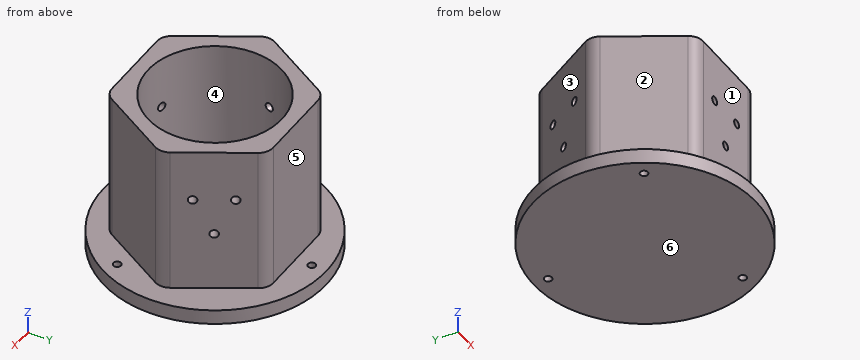
```python
from build123d import *

# Parameters (mm, degrees)
SKETCH1_R               = 75
BOSS_EXTRUDE1_DEPTH     = 10
BOSS_EXTRUDE2_DEPTH     = 100
SKETCH4_R               = 45
CUT_EXTRUDE1_DEPTH      = 100
CUT_EXTRUDE2_REACH      = 187.469
CUT_EXTRUDE2_END_RADIUS = 45
SKETCH5_R               = 2.8
CIRPATTERN1_COUNT       = 3
SKETCH7_R               = 2.55
CUT_EXTRUDE3_DEPTH      = 10


with BuildPart() as part:
    # Sketch1 → Boss-Extrude1 (new body)
    with BuildSketch(Plane.XY):
        Circle(SKETCH1_R)
    extrude(amount=BOSS_EXTRUDE1_DEPTH)

    # Sketch2 → Boss-Extrude2 (add)
    with BuildSketch(Plane.XY.offset(10)):
        with BuildLine():
            Line((59.613248654, 5), (34.136751346, 49.126587737))
            ThreePointArc((34.136751346, 49.126587737), (30.476497308, 52.786841774), (25.476497308, 54.126587737))
            Line((25.476497308, 54.126587737), (-25.476497308, 54.126587737))
            ThreePointArc((-25.476497308, 54.126587737), (-30.476497308, 52.786841774), (-34.136751346, 49.126587737))
            Line((-34.136751346, 49.126587737), (-59.613248654, 5))
            ThreePointArc((-59.613248654, 5), (-60.952994616, 0), (-59.613248654, -5))
            Line((-59.613248654, -5), (-34.136751346, -49.126587737))
            ThreePointArc((-34.136751346, -49.126587737), (-30.476497308, -52.786841774), (-25.476497308, -54.126587737))
            Line((-25.476497308, -54.126587737), (25.476497308, -54.126587737))
            ThreePointArc((25.476497308, -54.126587737), (30.476497308, -52.786841774), (34.136751346, -49.126587737))
            Line((34.136751346, -49.126587737), (59.613248654, -5))
            ThreePointArc((59.613248654, -5), (60.952994616, 0), (59.613248654, 5))
        make_face()
    extrude(amount=BOSS_EXTRUDE2_DEPTH)

    # Sketch4 → Cut-Extrude1 (cut)
    with BuildSketch(Plane.XY.offset(110)):
        Circle(SKETCH4_R)
    extrude(amount=-CUT_EXTRUDE1_DEPTH, mode=Mode.SUBTRACT)

    # Cut-Extrude2: up to this cylinder (the profile starts outside it)
    cut_extrude2_end = Plane(origin=(0, 0, 62.5), z_dir=(0, 0, 1)) * Cylinder(CUT_EXTRUDE2_END_RADIUS, 490.938, mode=Mode.PRIVATE)
    # Sketch5 → Cut-Extrude2 (cut, up to the surface)
    with BuildSketch(Plane.XZ.offset(54.126587737), mode=Mode.PRIVATE) as cut_extrude2_sk1:
        with Locations((0, 50)):
            Circle(SKETCH5_R)
    cut_extrude2_tool1 = extrude(cut_extrude2_sk1.sketch, amount=-CUT_EXTRUDE2_REACH, mode=Mode.PRIVATE) - cut_extrude2_end
    # Sketch5 → Cut-Extrude2 (cut, up to the surface)
    with BuildSketch(Plane.XZ.offset(54.126587737), mode=Mode.PRIVATE) as cut_extrude2_sk2:
        with Locations((-12.5, 75)):
            Circle(SKETCH5_R)
    cut_extrude2_tool2 = extrude(cut_extrude2_sk2.sketch, amount=-CUT_EXTRUDE2_REACH, mode=Mode.PRIVATE) - cut_extrude2_end
    # Sketch5 → Cut-Extrude2 (cut, up to the surface)
    with BuildSketch(Plane.XZ.offset(54.126587737), mode=Mode.PRIVATE) as cut_extrude2_sk3:
        with Locations((12.5, 75)):
            Circle(SKETCH5_R)
    cut_extrude2_tool3 = extrude(cut_extrude2_sk3.sketch, amount=-CUT_EXTRUDE2_REACH, mode=Mode.PRIVATE) - cut_extrude2_end
    cut_extrude2 = cut_extrude2_tool1.solids().sort_by_distance((0, -54.126588, 50))[0] + cut_extrude2_tool2.solids().sort_by_distance((-12.5, -54.126588, 75))[0] + cut_extrude2_tool3.solids().sort_by_distance((12.5, -54.126588, 75))[0]
    add(cut_extrude2, mode=Mode.SUBTRACT)

    # CirPattern1: Cut-Extrude2 ×3 about axis
    cirpattern1_axis = Axis((0, 0, -117.279220614), (0, 0, 1))
    for i in range(1, CIRPATTERN1_COUNT):
        add(cut_extrude2.rotate(cirpattern1_axis, i * 360 / CIRPATTERN1_COUNT), mode=Mode.SUBTRACT)

    # Sketch7 → Cut-Extrude3 (cut)
    with BuildSketch(Plane.XY.offset(10)):
        with Locations((0, 65)):
            Circle(SKETCH7_R)
        with Locations((56.291651246, -32.5)):
            Circle(SKETCH7_R)
        with Locations((-56.291651246, -32.5)):
            Circle(SKETCH7_R)
    extrude(amount=-CUT_EXTRUDE3_DEPTH, mode=Mode.SUBTRACT)


solid = part.part
```
Input: part model. Units: mm. Frame: model coordinates. Face numbers are marked on the shaded views. A direction names the side the tool comes from. Give positions to 0.01 mm unless a question says otherwise; leave off trailing zeros. Loops run counter-clockwise (first coordinate to the right, second up) from the corner with the lowest first, then second, coordinate; pieces in that order, holes last. Notation, with made-up numbers: M 4.25,78 L 49.25,78 A34 cw 49.25,113 Z; hole C 60.25,-19 d6. An arc over 180 degrees is marked long. Answer as CSV lines item,"result". Start each with the question number.
1. Section D-D on y = 0. Return loops of the section in (x, z), plus the area to 3 significant figures.
2. Section A-A on z = 83.5. Return loops of the section in (x, y).
3. Line query: L1, parallel to X at y = -49, z = 75; L2, parallel to Z at x = 12.5, y = -47.5; L3, parallel to Z at x = -31, y = -4. Output: solid intervals per line, ascending.
4. Pin query (flat end, axial travel): P1, Ø12, axis at x = 57.5, z = 88.5, coming from the +Y side; P2, Ø10, axis at x = 0, z = 72.5, coming from the -Y side; P3, Ø3, axis at x = -28.5, y = 54, coming from the +Z side; P4, Ø1.5, axis at x = 57, z = 97, coming from the -Y side. Return the tip coordinate at first contact, or that it passes through.
5. Reachability of the marked faces 1, 2 and 3 from +Z, -Z, +X, -X, +Y, -Y: full face, straight path, thin tool, end or side. Return the list, or none.
6. Pull-direction query (Y, two-part tool) for the marked faces 4, 5 and 6; classes: released by +Y, released by -Y, zero draft, split by the parting line, or undercut.
7. Section B-B on y = 65. Return loops of the section in (x, z), plus the area to 3 significant figures.
8. Section C-C on x = 0. Return loops of the section in (y, z).
Computed values:
1,outline,"M -75,0 L 75,0 L 75,10 L 60.95,10 L 60.95,110 L 45,110 L 45,10 L -45,10 L -45,110 L -60.95,110 L -60.95,10 L -75,10 Z"
1,area,"4,690 mm²"
2,outline,"M -59.61,-5 L -34.14,-49.13 A10 ccw -25.48,-54.13 L 25.48,-54.13 A10 ccw 34.14,-49.13 L 59.61,-5 A10 ccw 59.61,5 L 34.14,49.13 A10 ccw 25.48,54.13 L -25.48,54.13 A10 ccw -34.14,49.13 L -59.61,5 A10 ccw Z; hole C 0,0 d90"
3,L1,"x = -34.21 to -15.3, -9.7 to 9.7, 15.3 to 34.21"
3,L2,"z = 0 to 72.2, 77.8 to 110"
3,L3,"z = 0 to 10"
4,P1,"stops at y = 19.05"
4,P2,"stops at y = -54.13"
4,P3,"stops at z = 110"
4,P4,"stops at y = -10.83"
5,face 1,"+Z, +X, -X, -Y"
5,face 2,"+Z, -X, -Y"
5,face 3,"+Z, -X, +Y"
6,face 4,"undercut"
6,face 5,"released by +Y"
6,face 6,"zero draft"
7,outline,"M -37.42,0 L -2.55,0 L -2.55,10 L -37.42,10 Z; M 2.55,0 L 37.42,0 L 37.42,10 L 2.55,10 Z"
7,area,"697 mm²"
8,outline,"M -75,0 L 62.45,0 L 62.45,10 L 54.13,10 L 54.13,110 L 45,110 L 45,10 L -45,10 L -45,47.2 L -54.13,47.2 L -54.13,10 L -75,10 Z; M -54.13,52.8 L -45,52.8 L -45,110 L -54.13,110 Z; M 67.55,0 L 75,0 L 75,10 L 67.55,10 Z"
